Verification items for the finished model (mm, model axes). Face numbers are marked on the shaded views. Round coordinates to 2 decimals unless told otherwise and drop trailing zeros. Write each loop counter-clockwise with the first axis right and the second up, starting at its lowest first coordinate (ties: lowest second). Pieces come first, ordered by that corner, then holes. Notation, with made-up numbers: (-14.5, 63) -> (9.5, 63) arc R26 ccw to (9.5, 99) -> close; hole circle Ø9 at (-10, -40). An arc over 180 degrees is marked (long way). Use CSV: the item, a comma, the result in double quotes.
```python
from build123d import *

# Parameters (mm, degrees)
CYLINDER080_R      = 1.8
CYLINDER080_DEPTH  = 10
BOX406008008_W     = 19
BOX406008008_H     = 19
BOX406008008_DEPTH = 2
CHAMFER026_SIZE    = 0.5
CHAMFER027_SIZE    = 0.5


with BuildPart() as cylinder078:
    # Cylinder080 → Cylinder080 (new body)
    with BuildSketch(Plane.XY.offset(-4)):
        Circle(CYLINDER080_R)
    extrude(amount=CYLINDER080_DEPTH)


with BuildPart() as filler_plate:
    # Box406008008 → Box406008008 (new body)
    with BuildSketch(Plane(origin=(-9.5, -9.5, 0), x_dir=(1, 0, 0), z_dir=(0, 0, 1))):
        with Locations((9.5, 9.5)):
            Rectangle(BOX406008008_W, BOX406008008_H)
    extrude(amount=BOX406008008_DEPTH)

    # Cut173011013: cut Cylinder078
    add(cylinder078.part, mode=Mode.SUBTRACT)

    # Chamfer026
    chamfer026_edges = [filler_plate.edges().sort_by_distance(p)[0] for p in [
        (-1.8, 0, 2),
    ]]
    chamfer(chamfer026_edges, length=CHAMFER026_SIZE)

    # Chamfer027
    chamfer027_edges = [filler_plate.edges().sort_by_distance(p)[0] for p in [
        (-9.5, 0, 0),
        (0, 9.5, 0),
        (0, -9.5, 0),
        (9.5, 0, 0),
    ]]
    chamfer(chamfer027_edges, length=CHAMFER027_SIZE)


solid = filler_plate.part
```
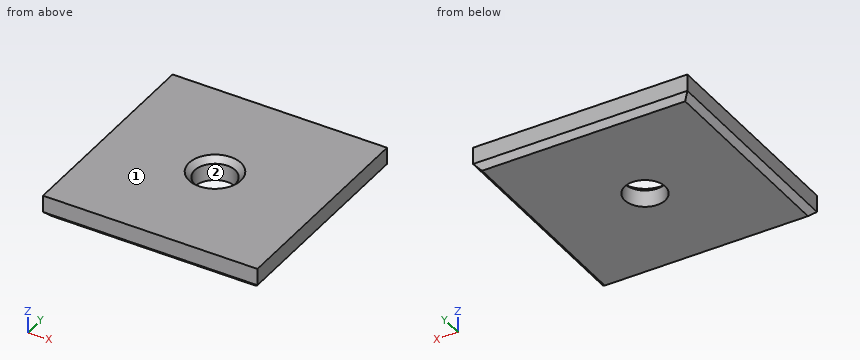
Q1. Mould release check, pull along X, two halves, no side actions. Record for the marked faces 1 and 2: released by +X, released by -X, zero draft, split by the parting line, or undercut.
Filled in:
face 1,"zero draft"
face 2,"undercut"
Q2. Go/stop test with a flat-tipped pin: P1, Ø2, axis at x = 0, y = 0, coming from the -Z side. Record where the tip stops, or that it passes through.
Filled in:
P1,"through"
Q3. Material ranges on L1, parallel to X at y = 0, z = 0.6; L2, parallel to Y at x = -1.25, z = 0.2, recorded low to high.
Filled in:
L1,"-9.5 to -1.8, 1.8 to 9.5"
L2,"-9.2 to -1.3, 1.3 to 9.2"
Q4. Section check A-A (x = 0). Record the cut outline in (y, z), plus the area to 3 significant figures.
Filled in:
outline,"(-9.5, 0.5) -> (-9, 0) -> (-1.8, 0) -> (-1.8, 1.5) -> (-2.3, 2) -> (-9.5, 2) -> close; (1.8, 0) -> (9, 0) -> (9.5, 0.5) -> (9.5, 2) -> (2.3, 2) -> (1.8, 1.5) -> close"
area,"30.3 mm²"
Q5. Section check C-C (z = 1). Record the cut outline in (x, y), plus the area to 3 significant figures.
Filled in:
outline,"(-9.5, -9.5) -> (9.5, -9.5) -> (9.5, 9.5) -> (-9.5, 9.5) -> close; hole circle Ø3.6 at (0, 0)"
area,"351 mm²"
